Input: part model. Units: mm. Frame: model coordinates. Round coordinates to 2 decimals unless told otherwise and drop trailing zeros. Order: outer loops, then holes, each group sorted by start corner. A loop starts at its lowest first (then second) coordinate and runs counter-clockwise, first axis right, second up. Notation, with made-up numbers: (82.25, 4.5) -> (133.25, 4.5) arc R14 cw to (133.25, 22.5) -> close; hole circle Ø1 at (9.25, 66). An arc over 180 degrees is marked (long way). Use a Markdown table: item, result.
from build123d import *
from build123d.topology import SkipClean

# Parameters (mm, degrees)
SKETCH1_R           = 0.635
BOSS_EXTRUDE1_DEPTH = 15.24
SKETCH2_R           = 0.635
BOSS_EXTRUDE2_DEPTH = 12.7
SKETCH3_R           = 0.635
BOSS_EXTRUDE3_DEPTH = 6.35


with BuildPart() as part:
    # Sketch1 → Boss-Extrude1 (new, symmetric)
    with BuildSketch(Plane.XY):
        Circle(SKETCH1_R)
    extrude(amount=BOSS_EXTRUDE1_DEPTH, both=True)

    # Sketch2 → Boss-Extrude2 (add)
    with BuildSketch(Plane(origin=(0, 0.635, 0), x_dir=(1, 0, 0), z_dir=(0, 1, 0))):
        with Locations(Location((0, -15.24, 0), (0, 0, 270))):
            Circle(SKETCH2_R)
    boss_extrude2 = extrude(amount=-BOSS_EXTRUDE2_DEPTH)

    # Sketch3 → Boss-Extrude3 (add)
    with SkipClean():  # the faces are left unmerged after this step: merging them gives an invalid solid
        with BuildSketch(Plane.XY.offset(15.875)):
            with Locations((0, -12.065)):
                Circle(SKETCH3_R)
        boss_extrude3 = extrude(amount=-BOSS_EXTRUDE3_DEPTH)

    # Mirror1: Boss-Extrude2, Boss-Extrude3 across plane
    with SkipClean():  # the faces are left unmerged after this step: merging them gives an invalid solid
        add(boss_extrude2.mirror(Plane.XY))
        add(boss_extrude3.mirror(Plane.XY))


solid = part.part
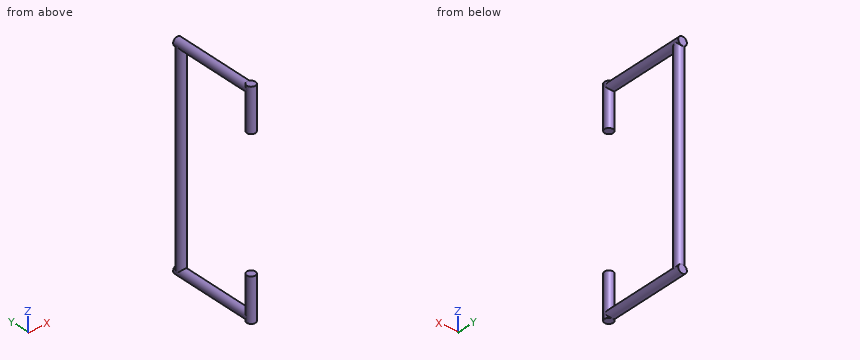
1) Cut plane B-B on x = 0.2. Return loops of the section in (y, z) (3 decimals).
Answer key:
| item | result |
|---|---|
| outline | (-12.668, -15.875) -> (-11.462, -15.875) -> (-11.462, -15.843) -> (0.635, -15.843) -> (0.635, -14.637) -> (0.603, -14.637) -> (0.603, 14.637) -> (0.635, 14.637) -> (0.635, 15.843) -> (-11.462, 15.843) -> (-11.462, 15.875) -> (-12.668, 15.875) -> (-12.668, 9.525) -> (-11.462, 9.525) -> (-11.462, 14.637) -> (-0.603, 14.637) -> (-0.603, -14.637) -> (-11.462, -14.637) -> (-11.462, -9.525) -> (-12.668, -9.525) -> close |
2) Cut plane A-A on z = 13. Return loops of the section in (x, y) (3 decimals).
Answer key:
| item | result |
|---|---|
| outline | circle Ø1.27 at (0, -12.065); circle Ø1.27 at (0, 0) |
3) Cut plane C-C on z = 7. Return loops of the section in (x, y) (3 decimals).
Answer key:
| item | result |
|---|---|
| outline | circle Ø1.27 at (0, 0) |
4) Ray query, probe 1 along Z at (x, y) = (-0.05, -11); probe 2 along Y at (x, z) = (0.05, 8); probe 3 along Z at (x, y) = (-0.5, -2). Return the intervals inside material, ascending.
Answer key:
| item | result |
|---|---|
| probe 1 | z = -15.87 to -14.61, 14.61 to 15.87 |
| probe 2 | y = -0.63 to 0.63 |
| probe 3 | z = -15.63 to -14.85, 14.85 to 15.63 |
